from build123d import *

# Parameters (mm, degrees)
F0_R     = 46.99
F1_DEPTH = 1.397
F3_DEPTH = 25.4
F4_R     = 6.35
F5_DEPTH = 7.62
F6_SIZE  = 0.508
F8_DEPTH = 20.32


with BuildPart() as f1:
    # F0 (on Top) → F1 (new body)
    with BuildSketch(Plane.XY):
        Circle(F0_R)
    extrude(amount=F1_DEPTH)

    # F2 (on face) → F3 (cut)
    with BuildSketch(Plane(origin=(0, 0, 0), x_dir=(1, 0, 0), z_dir=(0, 0, -1))):
        Polygon((2.4929984624, 4.318), (-2.4929984624, 4.318), (-4.9859969247, 0), (-2.4929984624, -4.318), (2.4929984624, -4.318), (4.9859969247, 0), align=None)
    extrude(amount=-F3_DEPTH, mode=Mode.SUBTRACT)

    # F4 (on face) → F5 (join)
    with BuildSketch(Plane.XY.offset(1.397)):
        Circle(F4_R)
        Polygon((2.4929984624, 4.318), (4.9859969247, 0), (2.4929984624, -4.318), (-2.4929984624, -4.318), (-4.9859969247, 0), (-2.4929984624, 4.318), align=None, mode=Mode.SUBTRACT)
    extrude(amount=F5_DEPTH)

    # F6
    f6_edges = [f1.edges().sort_by_distance(p)[0] for p in [
        (-6.35, 0, 9.017),
    ]]
    chamfer(f6_edges, length=F6_SIZE)

    # F7 (on face) → F8 (join)
    with BuildSketch(Plane.XY.offset(1.397)):
        with BuildLine():
            ThreePointArc((10.9985226281, 6.35), (17.5112017635, 26.1092350832), (10.6793059213, 45.7603816094))
            ThreePointArc((10.6793059213, 45.7603816094), (9.067413692, 46.1068553356), (7.4443589893, 46.396569046))
            ThreePointArc((7.4443589893, 46.396569046), (15.9253452898, 27.4252340455), (10.3083918417, 7.4180224884))
            Line((10.3083918417, 7.4180224884), (10.9985226281, 6.35))
        make_face()
        with BuildLine():
            ThreePointArc((12.7, 0), (28.2197631195, 13.8556599737), (32.1287410273, 34.29))
            ThreePointArc((32.1287410273, 34.29), (30.9060382717, 35.3960011633), (29.6452885226, 36.4584279476))
            ThreePointArc((29.6452885226, 36.4584279476), (27.5043706077, 15.7882767433), (12.6363404513, 1.27))
            Line((12.6363404513, 1.27), (12.7, 0))
        make_face()
        with BuildLine():
            ThreePointArc((44.9693059213, 13.6316405821), (44.4634148552, 15.2008170639), (43.9027869369, 16.7512805234))
            ThreePointArc((43.9027869369, 16.7512805234), (31.713622033, -0.0791365622), (11.5783918417, -5.2183179628))
            Line((11.5783918417, -5.2183179628), (10.9985226281, -6.35))
            ThreePointArc((10.9985226281, -6.35), (31.3668617372, -2.1105280363), (44.9693059213, 13.6316405821))
        make_face()
        with BuildLine():
            ThreePointArc((45.7603816094, -10.6793059213), (46.1068553356, -9.067413692), (46.396569046, -7.4443589893))
            ThreePointArc((46.396569046, -7.4443589893), (27.4252340455, -15.9253452898), (7.4180224884, -10.3083918417))
            Line((7.4180224884, -10.3083918417), (6.35, -10.9985226281))
            ThreePointArc((6.35, -10.9985226281), (26.1092350832, -17.5112017635), (45.7603816094, -10.6793059213))
        make_face()
        with BuildLine():
            ThreePointArc((34.29, -32.1287410273), (35.3960011633, -30.9060382717), (36.4584279476, -29.6452885226))
            ThreePointArc((36.4584279476, -29.6452885226), (15.7882767433, -27.5043706077), (1.27, -12.6363404513))
            Line((1.27, -12.6363404513), (0, -12.7))
            ThreePointArc((0, -12.7), (13.8556599737, -28.2197631195), (34.29, -32.1287410273))
        make_face()
        with BuildLine():
            ThreePointArc((13.6316405821, -44.9693059213), (15.2008170639, -44.4634148552), (16.7512805234, -43.9027869369))
            ThreePointArc((16.7512805234, -43.9027869369), (-0.0791365622, -31.713622033), (-5.2183179628, -11.5783918417))
            Line((-5.2183179628, -11.5783918417), (-6.35, -10.9985226281))
            ThreePointArc((-6.35, -10.9985226281), (-2.1105280363, -31.3668617372), (13.6316405821, -44.9693059213))
        make_face()
        with BuildLine():
            ThreePointArc((-10.6793059213, -45.7603816094), (-9.067413692, -46.1068553356), (-7.4443589893, -46.396569046))
            ThreePointArc((-7.4443589893, -46.396569046), (-15.9253452898, -27.4252340455), (-10.3083918417, -7.4180224884))
            Line((-10.3083918417, -7.4180224884), (-10.9985226281, -6.35))
            ThreePointArc((-10.9985226281, -6.35), (-17.5112017635, -26.1092350832), (-10.6793059213, -45.7603816094))
        make_face()
        with BuildLine():
            ThreePointArc((-32.1287410273, -34.29), (-30.9060382717, -35.3960011633), (-29.6452885226, -36.4584279476))
            ThreePointArc((-29.6452885226, -36.4584279476), (-27.5043706077, -15.7882767433), (-12.6363404513, -1.27))
            Line((-12.6363404513, -1.27), (-12.7, 0))
            ThreePointArc((-12.7, 0), (-28.2197631195, -13.8556599737), (-32.1287410273, -34.29))
        make_face()
        with BuildLine():
            ThreePointArc((-10.9985226281, 6.35), (-31.3668617372, 2.1105280363), (-44.9693059213, -13.6316405821))
            ThreePointArc((-44.9693059213, -13.6316405821), (-44.4634148552, -15.2008170639), (-43.9027869369, -16.7512805234))
            ThreePointArc((-43.9027869369, -16.7512805234), (-31.713622033, 0.0791365622), (-11.5783918417, 5.2183179628))
            Line((-11.5783918417, 5.2183179628), (-10.9985226281, 6.35))
        make_face()
        with BuildLine():
            ThreePointArc((-6.35, 10.9985226281), (-26.1092350832, 17.5112017635), (-45.7603816094, 10.6793059213))
            ThreePointArc((-45.7603816094, 10.6793059213), (-46.1068553356, 9.067413692), (-46.396569046, 7.4443589893))
            ThreePointArc((-46.396569046, 7.4443589893), (-27.4252340455, 15.9253452898), (-7.4180224884, 10.3083918417))
            Line((-7.4180224884, 10.3083918417), (-6.35, 10.9985226281))
        make_face()
        with BuildLine():
            ThreePointArc((0, 12.7), (-13.8556599737, 28.2197631195), (-34.29, 32.1287410273))
            ThreePointArc((-34.29, 32.1287410273), (-35.3960011633, 30.9060382717), (-36.4584279476, 29.6452885226))
            ThreePointArc((-36.4584279476, 29.6452885226), (-15.7882767433, 27.5043706077), (-1.27, 12.6363404513))
            Line((-1.27, 12.6363404513), (0, 12.7))
        make_face()
        with BuildLine():
            ThreePointArc((6.35, 10.9985226281), (2.1105280363, 31.3668617372), (-13.6316405821, 44.9693059213))
            ThreePointArc((-13.6316405821, 44.9693059213), (-15.2008170639, 44.4634148552), (-16.7512805234, 43.9027869369))
            ThreePointArc((-16.7512805234, 43.9027869369), (0.0791365622, 31.713622033), (5.2183179628, 11.5783918417))
            Line((5.2183179628, 11.5783918417), (6.35, 10.9985226281))
        make_face()
    extrude(amount=F8_DEPTH)


solid = f1.part
Part model, mm, in its own coordinate system. A direction names the side the tool comes from. Round coordinates to 2 decimals unless told otherwise and drop trailing zeros. Loops run counter-clockwise (first coordinate to the right, second up) from the corner with the lowest first, then second, coordinate; pieces in that order, holes last. Notation, with made-up numbers: (-35, -14) - (12, -14) arc R27 ccw to (12, 10) - close; hole circle Ø9 at (36, -22). An arc over 180 degrees is marked (long way). Answer as a JSON object with one key per item and string values.
Item 1: Band-saw the part on D-D on y = 26. List the corners of the cut face in (x, z).
Output:
{"outline": "(-39.14, 0) - (39.14, 0) - (39.14, 1.4) - (32.21, 1.4) - (32.21, 21.72) - (30.39, 21.72) - (30.39, 1.4) - (17.51, 1.4) - (17.51, 21.72) - (16, 21.72) - (16, 1.4) - (4.64, 1.4) - (4.64, 21.72) - (3.13, 21.72) - (3.13, 1.4) - (-10.45, 1.4) - (-10.45, 21.72) - (-13.04, 21.72) - (-13.04, 1.4) - (-39.14, 1.4) - close"}
Item 2: Pin check, flat tips, straight feed: pin 1 (12 mm diameter, centred on x = 15.5, z = 16, fed in from +Y); pin 2 (4 mm diameter, centred on x = 0.5, z = 3, fed in from +Y); pin 3 (1.5 mm diameter, centred on y = -32.5, z = 9, fed in from -X). Stop position of each tip, or through.
Output:
{"pin 1": "y = 46.02", "pin 2": "y = 46.99", "pin 3": "x = -32.38"}
Item 3: Pull direction X, two halves, no side cores. Call faces 1 (the face through (2.26, 31.11, 11.41)), 2 (the face through (0, 33, 21.717)), 3 (the face through (0, 4.318, 4)): pulls with the +X half, pulls with the -X half, needs draft (parallel to the pull), parting line crosses it, or undercut.
Output:
{"face 1": "undercut", "face 2": "needs draft", "face 3": "undercut"}
Item 4: Band-saw the part on C-C on z = 18.25. State how many separate pieces and enclosed holes the cut face has, plus the area to 3 significant figures.
Output:
{"separate pieces": "12", "enclosed holes": "0", "area": "792 mm2"}
Item 5: Band-saw the part on B-B on x = -38. List the corners of the cut face in (y, z), plus the area to 3 significant figures.
Output:
{"outline": "(-27.64, 0) - (27.64, 0) - (27.64, 1.4) - (15.15, 1.4) - (15.15, 21.72) - (13.19, 21.72) - (13.19, 1.4) - (-3.06, 1.4) - (-3.06, 21.72) - (-5.62, 21.72) - (-5.62, 1.4) - (-27.64, 1.4) - close", "area": "169 mm2"}
Item 6: Band-saw the part on A-A on y = -19. List the corners of the cut face in (x, z), plus the area to 3 significant figures.
Output:
{"outline": "(-42.98, 0) - (42.98, 0) - (42.98, 1.4) - (5.16, 1.4) - (5.16, 21.72) - (3.56, 21.72) - (3.56, 1.4) - (-5.04, 1.4) - (-5.04, 21.72) - (-6.33, 21.72) - (-6.33, 1.4) - (-15.37, 1.4) - (-15.37, 21.72) - (-16.78, 21.72) - (-16.78, 1.4) - (-28.84, 1.4) - (-28.84, 21.72) - (-30.57, 21.72) - (-30.57, 1.4) - (-42.98, 1.4) - close", "area": "243 mm2"}
Item 7: Tool access for faces 4 (the face through (16.8, -28.4, 21.717)), 5 (the face through (-3.757, 2.129, 4.445)), 6 (the face through (-16.056, 27.632, 11.415)): list every direction of +Z, -Z, +X, -X, +Y, -Y with a clear straight run to the whole face (end or side of a thin tool).
Output:
{"face 4": "+Z, +X, -X, +Y, -Y", "face 5": "+Z, -Z", "face 6": "+Z"}
Item 8: Wall check: L1, parallel to Y at x = 34.5, z = 6.5; L2, parallel to Y at x = 27.5, z = 10.5; L3, parallel to Y at x = 24.5, z = 6.75. Give the ranges that are in metal, low to high.
Output:
{"L1": "-31.9 to -30.06, -16.34 to -14.55, -0.01 to 2.06", "L2": "-32.35 to -30.51, -17.47 to -15.92, -4.05 to -2.48, 12.65 to 15.78", "L3": "-31.99 to -30.2, -17.48 to -16, -5.14 to -3.69, 8.59 to 10.83"}
